from build123d import *

# Parameters (mm, degrees)
SKETCH_2_R      = 25.625
EXTRUDE_1_DEPTH = 21.5
EXTRUDE_2_DEPTH = 7.5


with BuildPart() as part:
    # 草圖2 → 伸長1 (new body)
    with BuildSketch(Plane(origin=(0, 0, 0), x_dir=(0, 0, -1), z_dir=(1, 0, 0))):
        Circle(SKETCH_2_R)
    extrude(amount=EXTRUDE_1_DEPTH)

    # 草圖3 → 伸長2 (add)
    with BuildSketch(Plane(origin=(21.5, 0, 0), x_dir=(0, 0, -1), z_dir=(1, 0, 0))):
        Polygon((0, 20.784609691), (-18, 10.392304845), (-18, -10.392304845), (0, -20.784609691), (18, -10.392304845), (18, 10.392304845), align=None)
    extrude(amount=EXTRUDE_2_DEPTH)

    # 草圖4 → 除料-旋轉1 (revolve, cut)
    with BuildSketch(Plane.XY):
        Polygon((27.392304845, 20.784609691), (29, 20.784609691), (29, 18), align=None)
    revolve(axis=Axis((0, 0, 0), (1, 0, 0)), mode=Mode.SUBTRACT)

    # 草圖5 → 除料-旋轉2 (revolve, cut)
    with BuildSketch(Plane.XY, mode=Mode.PRIVATE) as cut_revolve_2_sk:
        Polygon((0, 0), (0, 21.5), (10.5, 21.5), (10.5, 23), (16.5, 23), (16.5, 16.5), (29, 16.5), (29, 0), align=None)
    revolve(cut_revolve_2_sk.sketch.rotate(Axis((0, 0, 0), (1, 0, 0)), 90), axis=Axis((0, 0, 0), (1, 0, 0)), mode=Mode.SUBTRACT)


solid = part.part
Design review of the part built by this model. Coordinates are the model's own, in mm. A direction names the side the tool comes from. Round coordinates to 2 decimals unless told otherwise and drop trailing zeros. Loops run counter-clockwise (first coordinate to the right, second up) from the corner with the lowest first, then second, coordinate; pieces in that order, holes last. Notation, with made-up numbers: M 18.25,36 L 40.25,36 A30 cw 40.25,75 Z; hole C 22.5,59 d2. An arc over 180 degrees is marked long. Answer as a JSON object with one key per item and string values.
Item 1: Wall thickness on L1, parallel to Y at x = 12.9, z = 0 (3 decimals); L2, parallel to X at y = 8, z = 21; L3, parallel to Y at x = 5, z = 0 (3 decimals): over which ranges is each line inside the solid? List them lowest first. Write a range as from..to.
Answer sheet:
{"L1": "y = -25.625..-23, 23..25.625", "L2": "x = 0..10.5, 16.5..21.5", "L3": "y = -25.625..-21.5, 21.5..25.625"}
Item 2: We need section A-A on x = 25.25. Give the boundary of the cut face in (y, z), and give its area (3 significant figures).
Answer sheet:
{"outline": "M -20.78,0 L -10.39,-18 L 10.39,-18 L 20.78,0 L 10.39,18 L -10.39,18 Z; hole C 0,0 d33", "area": "267 mm^2"}
Item 3: We need section C-C on x = 18.5. Give the boundary of the cut face in (y, z) (3 decimals), and give its area (3 significant figures).
Answer sheet:
{"outline": "C 0,0 d51.25; hole C 0,0 d33", "area": "1,210 mm^2"}
Item 4: Clearance check with flat-ended pins moving along their axes: P1, Ø4, axis at x = 21.5, z = 10, coming from the +Y side; P2, Ø1.5, axis at x = 11.5, z = 10.5, coming from the -Y side; P3, Ø6, axis at x = 19.5, y = 5, coming from the -Z side; P4, Ø10, axis at y = 13, z = 19.5, coming from the -X side. State where each tip first meets the part, or that it passes through.
Answer sheet:
{"P1": "stops at y = 24.34", "P2": "stops at y = -23.7", "P3": "stops at z = -25.55", "P4": "stops at x = 0"}
Item 5: We need section B-B on x = 7. Give the boundary of the cut face in (y, z) (3 decimals).
Answer sheet:
{"outline": "C 0,0 d51.25; hole C 0,0 d43"}
Item 6: The part is to be moulded in two halves that separate along Y. For faces 1 (the flat face through (0, 21, 6)), 2 (the flat face through (25.198, 15.661, 8.874)), 3 (the flat face through (16.5, -5, -16)), say which applies: pulls with the +Y half, pulls with the -Y half, needs draft (parallel to the pull), parting line crosses it, or undercut.
Answer sheet:
{"face 1": "needs draft", "face 2": "pulls with the +Y half", "face 3": "undercut"}
Item 7: Machinability: for faces 4 (the flat face through (10.5, 14, -17)), 5 (the flat face through (25, 0, -18)), 6 (the cylindrical face through (5.324, -21.317, -2.799)), 7 (the flat face through (25.198, 15.516, -9.126)), which of the approach directions +Z, -Z, +X, -X, +Y, -Y give a long, thin tool a straight path to every point of the face, cutting with its end or side? Answer none if there is none.
Answer sheet:
{"face 4": "none", "face 5": "-Z, +X, +Y, -Y", "face 6": "-X", "face 7": "-Z, +X, +Y"}
